Here's how the part is built. I have some questions about the finished solid (model axes, mm). Round coordinates to 2 decimals unless told otherwise and drop trailing zeros. Order: outer loops, then holes, each group sorted by start corner. A loop starts at its lowest first (then second) coordinate and runs counter-clockwise, first axis right, second up. Notation, with made-up numbers: (17.5, -26) -> (45.5, -26) arc R12 cw to (45.5, -12) -> close; hole circle Ø11 at (44, -15). An arc over 180 degrees is marked (long way). One line per item, written item: value.
```python
from build123d import *

# Parameters (mm, degrees)
SKETCH1_W           = 750
SKETCH1_H           = 300
BOSS_EXTRUDE1_DEPTH = 10
SKETCH4_W           = 9.6
SKETCH4_H           = 49.5
SKETCH4_W_2         = 49.5
SKETCH4_H_2         = 9.6
CUT_EXTRUDE3_DEPTH  = 11
FILLET1_R           = 10


with BuildPart() as part:
    # Sketch1 → Boss-Extrude1 (new body)
    with BuildSketch(Plane(origin=(0, 0, 0), x_dir=(1, 0, 0), z_dir=(0, 1, 0))):
        with Locations((375, 150)):
            Rectangle(SKETCH1_W, SKETCH1_H)
    extrude(amount=BOSS_EXTRUDE1_DEPTH)

    # Sketch4 → Cut-Extrude3 (cut, through all)
    with BuildSketch(Plane(origin=(0, 10, 0), x_dir=(1, 0, 0), z_dir=(0, 1, 0))):
        with Locations((12.8, 100)):
            Rectangle(SKETCH4_W, SKETCH4_H)
        with Locations((12.8, 200)):
            Rectangle(SKETCH4_W, SKETCH4_H)
        with Locations((737.2, 200)):
            Rectangle(SKETCH4_W, SKETCH4_H)
        with Locations((737.2, 100)):
            Rectangle(SKETCH4_W, SKETCH4_H)
        with Locations((144.75, 287.2)):
            Rectangle(SKETCH4_W_2, SKETCH4_H_2)
        with Locations((244.75, 287.2)):
            Rectangle(SKETCH4_W_2, SKETCH4_H_2)
        with Locations((505.25, 287.2)):
            Rectangle(SKETCH4_W_2, SKETCH4_H_2)
        with Locations((605.25, 287.2)):
            Rectangle(SKETCH4_W_2, SKETCH4_H_2)
        with Locations((605.25, 12.8)):
            Rectangle(SKETCH4_W_2, SKETCH4_H_2)
        with Locations((505.25, 12.8)):
            Rectangle(SKETCH4_W_2, SKETCH4_H_2)
        with Locations((244.75, 12.8)):
            Rectangle(SKETCH4_W_2, SKETCH4_H_2)
        with Locations((144.75, 12.8)):
            Rectangle(SKETCH4_W_2, SKETCH4_H_2)
    extrude(amount=-CUT_EXTRUDE3_DEPTH, mode=Mode.SUBTRACT)

    # Fillet1
    fillet1_edges = [part.edges().sort_by_distance(p)[0] for p in [
        (0, 5, 0),
        (750, 5, 0),
        (750, 5, -300),
        (0, 5, -300),
    ]]
    fillet(fillet1_edges, radius=FILLET1_R)


solid = part.part
```
Q1. I need wall thicknesses on line 1 along X through (y, z) = (1.5, -83); line 2 along X through (y, z) = (9, -286); line 3 along Z through (x, y) = (234, 5). Which ranges of each line are inside material? Lowest first, please.
Answers:
line 1: 0 to 8, 17.6 to 732.4, 742 to 750
line 2: 0 to 120, 169.5 to 220, 269.5 to 480.5, 530 to 580.5, 630 to 750
line 3: -300 to -292, -282.4 to -17.6, -8 to 0
Q2. I want a section at A-A on z = -204.5. Write out the boundary of the cut face in (x, y), then the cut area to 3 significant figures.
Answers:
outline: (0, 0) -> (8, 0) -> (8, 10) -> (0, 10) -> close; (17.6, 0) -> (732.4, 0) -> (732.4, 10) -> (17.6, 10) -> close; (742, 0) -> (750, 0) -> (750, 10) -> (742, 10) -> close
area: 7,310 mm2
Q3. I want a section at B-B on y = 6.75. Give the number of separate pieces and of enclosed holes in the cut face, then the cut area to 3 significant figures.
Answers:
separate pieces: 1
enclosed holes: 12
area: 219,000 mm2
